Check sheet for the modelled part. Datum: model origin and axes. Units: mm. A direction names the side the tool comes from. Give positions to 0.01 mm unless a question says otherwise; leave off trailing zeros. Loops run counter-clockwise (first coordinate to the right, second up) from the corner with the lowest first, then second, coordinate; pieces in that order, holes last.
```python
from build123d import *

# Parameters (mm, degrees)
SKETCH1_W           = 104.5
SKETCH1_H           = 125.5
BOSS_EXTRUDE1_DEPTH = 4
FILLET1_R           = 5.25
EXTRUDE_THIN1_START = 11
EXTRUDE_THIN1_DEPTH = 11
CUT_EXTRUDE2_REACH  = 138.387
SKETCH6_R           = 1.5
SKETCH8_W           = 10
SKETCH8_H           = 11
BOSS_EXTRUDE2_DEPTH = 4.5
CHAMFER2_SIZE       = 4.5
SKETCH5_R           = 1.9
CUT_EXTRUDE3_DEPTH  = 164.998475603
SKETCH10_R          = 2.45
CUT_EXTRUDE4_DEPTH  = 5
SKETCH2_R           = 5.5
BOSS_EXTRUDE3_DEPTH = 8
CUT_EXTRUDE5_DEPTH  = 137.386628743
SKETCH13_R          = 1.75
CUT_EXTRUDE6_DEPTH  = 137.386628743
CHAMFER3_SIZE       = 4
SKETCH14_R          = 1.75
CUT_EXTRUDE7_DEPTH  = 137.386628743


with BuildPart() as part:
    # Sketch1 → Boss-Extrude1 (new body)
    with BuildSketch(Plane(origin=(0, 0, 0), x_dir=(1, 0, 0), z_dir=(0, 1, 0))):
        with Locations((0, 62.75)):
            Rectangle(SKETCH1_W, SKETCH1_H)
    extrude(amount=BOSS_EXTRUDE1_DEPTH)

    # Fillet1
    fillet1_edges = [part.edges().sort_by_distance(p)[0] for p in [
        (-52.25, 2, -125.5),
        (52.25, 2, -125.5),
        (52.25, 2, 0),
        (-52.25, 2, 0),
    ]]
    fillet(fillet1_edges, radius=FILLET1_R)

    # Sketch3 → Extrude-Thin1 (add)
    with BuildSketch(Plane(origin=(0, 4, 0), x_dir=(1, 0, 0), z_dir=(0, 1, 0)).offset(EXTRUDE_THIN1_START)):
        with BuildLine():
            Line((47, 125.5), (-47, 125.5))
            ThreePointArc((-47, 125.5), (-50.712310601, 123.962310601), (-52.25, 120.25))
            Line((-52.25, 120.25), (-52.25, 5.25))
            ThreePointArc((-52.25, 5.25), (-50.712310601, 1.537689399), (-47, 0))
            Line((-47, 0), (47, 0))
            ThreePointArc((47, 0), (50.712310601, 1.537689399), (52.25, 5.25))
            Line((52.25, 5.25), (52.25, 120.25))
            ThreePointArc((52.25, 120.25), (50.712310601, 123.962310601), (47, 125.5))
        make_face()
        with BuildLine():
            Line((47, 122.5), (-47, 122.5))
            ThreePointArc((-47, 122.5), (-48.590990258, 121.840990258), (-49.25, 120.25))
            Line((-49.25, 120.25), (-49.25, 5.25))
            ThreePointArc((-49.25, 5.25), (-48.590990258, 3.659009742), (-47, 3))
            Line((-47, 3), (47, 3))
            ThreePointArc((47, 3), (48.590990258, 3.659009742), (49.25, 5.25))
            Line((49.25, 5.25), (49.25, 120.25))
            ThreePointArc((49.25, 120.25), (48.590990258, 121.840990258), (47, 122.5))
        make_face(mode=Mode.SUBTRACT)
    extrude(amount=-EXTRUDE_THIN1_DEPTH)

    # Sketch6 → Cut-Extrude2 (cut, up to next)
    with BuildSketch(Plane(origin=(0, 4, 0), x_dir=(1, 0, 0), z_dir=(0, 1, 0)), mode=Mode.PRIVATE) as cut_extrude2_sk1:
        with Locations(Location((-37.5, 110.75, 0), (0, 0, 270))):
            Circle(SKETCH6_R)
    cut_extrude2_tool1 = extrude(cut_extrude2_sk1.sketch, amount=-CUT_EXTRUDE2_REACH, mode=Mode.PRIVATE) & part.part
    # Sketch6 → Cut-Extrude2 (cut, up to next)
    with BuildSketch(Plane(origin=(0, 4, 0), x_dir=(1, 0, 0), z_dir=(0, 1, 0)), mode=Mode.PRIVATE) as cut_extrude2_sk2:
        with Locations(Location((37.5, 110.75, 0), (0, 0, 270))):
            Circle(SKETCH6_R)
    cut_extrude2_tool2 = extrude(cut_extrude2_sk2.sketch, amount=-CUT_EXTRUDE2_REACH, mode=Mode.PRIVATE) & part.part
    # Sketch6 → Cut-Extrude2 (cut, up to next)
    with BuildSketch(Plane(origin=(0, 4, 0), x_dir=(1, 0, 0), z_dir=(0, 1, 0)), mode=Mode.PRIVATE) as cut_extrude2_sk3:
        with Locations(Location((37.5, 35.75, 0), (0, 0, 270))):
            Circle(SKETCH6_R)
    cut_extrude2_tool3 = extrude(cut_extrude2_sk3.sketch, amount=-CUT_EXTRUDE2_REACH, mode=Mode.PRIVATE) & part.part
    # Sketch6 → Cut-Extrude2 (cut, up to next)
    with BuildSketch(Plane(origin=(0, 4, 0), x_dir=(1, 0, 0), z_dir=(0, 1, 0)), mode=Mode.PRIVATE) as cut_extrude2_sk4:
        with Locations(Location((-37.5, 35.75, 0), (0, 0, 270))):
            Circle(SKETCH6_R)
    cut_extrude2_tool4 = extrude(cut_extrude2_sk4.sketch, amount=-CUT_EXTRUDE2_REACH, mode=Mode.PRIVATE) & part.part
    add(cut_extrude2_tool1.solids().sort_by_distance((-37.5, 4, -110.75))[0], mode=Mode.SUBTRACT)
    add(cut_extrude2_tool2.solids().sort_by_distance((37.5, 4, -110.75))[0], mode=Mode.SUBTRACT)
    add(cut_extrude2_tool3.solids().sort_by_distance((37.5, 4, -35.75))[0], mode=Mode.SUBTRACT)
    add(cut_extrude2_tool4.solids().sort_by_distance((-37.5, 4, -35.75))[0], mode=Mode.SUBTRACT)

    # Sketch8 → Boss-Extrude2 (add)
    with BuildSketch(Plane(origin=(-49.25, 0, 0), x_dir=(0, 0, -1), z_dir=(1, 0, 0))):
        with Locations((28.55, 9.5)):
            Rectangle(SKETCH8_W, SKETCH8_H)
        with Locations((108.55, 9.5)):
            Rectangle(SKETCH8_W, SKETCH8_H)
    boss_extrude2 = extrude(amount=BOSS_EXTRUDE2_DEPTH)

    # Mirror4: Boss-Extrude2 across plane
    add(boss_extrude2.mirror(Plane(origin=(0, 0, 0), x_dir=(0, 0, 1), z_dir=(1, 0, 0))))

    # Chamfer2
    chamfer2_edges = [part.edges().sort_by_distance(p)[0] for p in [
        (-49.25, 9.5, -113.55),
        (-49.25, 9.5, -103.55),
        (-49.25, 9.5, -33.55),
        (-49.25, 9.5, -23.55),
        (49.25, 9.5, -113.55),
        (49.25, 9.5, -103.55),
        (49.25, 9.5, -23.55),
        (49.25, 9.5, -33.55),
    ]]
    chamfer(chamfer2_edges, length=CHAMFER2_SIZE - 0.0001)  # a hair under: the kernel refuses the full size

    # Sketch5 → Cut-Extrude3 (cut, through all)
    with BuildSketch(Plane.ZY.offset(52.25)):
        with Locations((-108.55, 10)):
            Circle(SKETCH5_R)
        with Locations((-28.55, 10)):
            Circle(SKETCH5_R)
    extrude(amount=-CUT_EXTRUDE3_DEPTH, mode=Mode.SUBTRACT)

    # Sketch10 → Cut-Extrude4 (cut)
    with BuildSketch(Plane(origin=(-44.75, 0, 0), x_dir=(0, 0, -1), z_dir=(1, 0, 0))):
        with Locations((28.55, 10)):
            Circle(SKETCH10_R)
        with Locations((108.55, 10)):
            Circle(SKETCH10_R)
    cut_extrude4 = extrude(amount=-CUT_EXTRUDE4_DEPTH, mode=Mode.SUBTRACT)

    # Sketch2 → Boss-Extrude3 (add)
    with BuildSketch(Plane.XZ):
        with Locations(Location((-37.5, -14.75, 0), (0, 0, 90))):
            Circle(SKETCH2_R)
        with Locations(Location((37.5, -14.75, 0), (0, 0, 90))):
            Circle(SKETCH2_R)
        with Locations(Location((-22.5, -110.5, 0), (0, 0, 90))):
            Circle(SKETCH2_R)
        with Locations(Location((22.5, -110.5, 0), (0, 0, 90))):
            Circle(SKETCH2_R)
    extrude(amount=-BOSS_EXTRUDE3_DEPTH)

    # Sketch12 → Cut-Extrude5 (cut, through all)
    with BuildSketch(Plane(origin=(0, 4, 0), x_dir=(1, 0, 0), z_dir=(0, 1, 0))):
        Polygon((-34.324573519, 14.75), (-35.91228676, 17.5), (-39.08771324, 17.5), (-40.675426481, 14.75), (-39.08771324, 12), (-35.91228676, 12), align=None)
        Polygon((35.91228676, 12), (34.324573519, 14.75), (35.91228676, 17.5), (39.08771324, 17.5), (40.675426481, 14.75), (39.08771324, 12), align=None)
        Polygon((25.675426481, 110.5), (24.08771324, 107.75), (20.91228676, 107.75), (19.324573519, 110.5), (20.91228676, 113.25), (24.08771324, 113.25), align=None)
        Polygon((-19.324573519, 110.5), (-20.91228676, 113.25), (-24.08771324, 113.25), (-25.675426481, 110.5), (-24.08771324, 107.75), (-20.91228676, 107.75), align=None)
    extrude(amount=CUT_EXTRUDE5_DEPTH, mode=Mode.SUBTRACT)

    # Sketch13 → Cut-Extrude6 (cut, through all)
    with BuildSketch(Plane(origin=(0, 4, 0), x_dir=(1, 0, 0), z_dir=(0, 1, 0))):
        with Locations(Location((37.5, 14.75, 0), (0, 0, 270))):
            Circle(SKETCH13_R)
        with Locations(Location((-37.5, 14.75, 0), (0, 0, 270))):
            Circle(SKETCH13_R)
        with Locations(Location((-22.5, 110.5, 0), (0, 0, 270))):
            Circle(SKETCH13_R)
        with Locations(Location((22.5, 110.5, 0), (0, 0, 270))):
            Circle(SKETCH13_R)
    extrude(amount=-CUT_EXTRUDE6_DEPTH, mode=Mode.SUBTRACT)

    # Chamfer3
    chamfer3_edges = [part.edges().sort_by_distance(p)[0] for p in [
        (-37.5, 4, -20.25),
        (37.5, 4, -20.25),
    ]]
    chamfer(chamfer3_edges, length=CHAMFER3_SIZE - 0.0001)  # a hair under: the kernel refuses the full size

    # Sketch14 → Cut-Extrude7 (cut, through all)
    with BuildSketch(Plane(origin=(0, 4, 0), x_dir=(1, 0, 0), z_dir=(0, 1, 0))):
        with Locations(Location((-42.25, 96.25, 0), (0, 0, 270))):
            Circle(SKETCH14_R)
        with Locations(Location((19.75, 96.25, 0), (0, 0, 270))):
            Circle(SKETCH14_R)
        with Locations(Location((19.75, 44.25, 0), (0, 0, 270))):
            Circle(SKETCH14_R)
        with Locations(Location((-42.25, 44.25, 0), (0, 0, 270))):
            Circle(SKETCH14_R)
    extrude(amount=-CUT_EXTRUDE7_DEPTH, mode=Mode.SUBTRACT)

    # Mirror5: Cut-Extrude4 across plane
    add(cut_extrude4.mirror(Plane(origin=(0, 0, 0), x_dir=(0, 0, 1), z_dir=(1, 0, 0))), mode=Mode.SUBTRACT)


solid = part.part
```
(1) Access from +Z, -Z, +X, -X, +Y, -Y to the whole of each face (thin tool, end or side, straight path). Record for faces 4 (the face through (-1, 0, -64)), 5 (the face through (44.75, 7, -28)).
(2) Section check A-A on x = 37.5. Give the number of separate pieces and of enclosed holes in the cut face, plus the area to 3 significant figures.
(3) Section check C-C on x = -22.5. Record the boundary of the cut face in (y, z), plus the area to 3 significant figures.
(4) Section check B-B on z = -28.55. Record the boundary of the cut face in (x, y).
(5) Section check D-D on x = -10.5. Record the boundary of the cut face in (y, z), plus the area to 3 significant figures.
(6) Material ranges on line 1 (Z direction, x = 22.5, y = 6.25); line 2 (X direction, y = 1.85, z = -44.25); line 3 (X direction, y = 0.9, z = -110.5), recorded low to high.
(7) Release check for a two-part mould opening along Y. For faces 1 (the face through (51, 8.3, -27.7)), 2 (the face through (-49.25, 10, -69)), 3 (the face through (-36, 4, -16)) record: pulls with the +Y half, pulls with the -Y half, needs draft (parallel to the pull), parting line crosses it, or undercut.
(8) Gauge pin test, flat ends, axial feed: pin 1 Ø1 at (x, z) = (-40.5, -46.5) entering from -Y; pin 2 Ø3 at (x, z) = (17, -45) entering from +Y. Record the tip position at first contact, or that the pin passes through.
Computed values:
1. face 4: +Z, -Z, +X, -X, -Y
1. face 5: +Y
2. separate pieces: 4
2. enclosed holes: 0
2. area: 568 mm2
3. outline: (0, -125.5) - (15, -125.5) - (15, -122.5) - (4, -122.5) - (4, -116) - (8, -116) - (8, -113.25) - (4, -113.25) - (4, -112.25) - (0, -112.25) - close; (0, -108.75) - (4, -108.75) - (4, -107.75) - (8, -107.75) - (8, -105) - (4, -105) - (4, -3) - (15, -3) - (15, 0) - (0, 0) - close
3. area: 576 mm2
4. outline: (-52.25, 0) - (52.25, 0) - (52.25, 8.1) - (49.75, 8.1) - (49.75, 7.55) - (44.75, 7.55) - (44.75, 4) - (-44.75, 4) - (-44.75, 7.55) - (-49.75, 7.55) - (-49.75, 8.1) - (-52.25, 8.1) - close; (-52.25, 11.9) - (-49.75, 11.9) - (-49.75, 12.45) - (-44.75, 12.45) - (-44.75, 15) - (-52.25, 15) - close; (44.75, 12.45) - (49.75, 12.45) - (49.75, 11.9) - (52.25, 11.9) - (52.25, 15) - (44.75, 15) - close
5. outline: (0, -125.5) - (15, -125.5) - (15, -122.5) - (4, -122.5) - (4, -3) - (15, -3) - (15, 0) - (0, 0) - close
5. area: 568 mm2
6. line 1: z = -125.5 to -122.5, -116 to -113.25, -107.75 to -105, -3 to 0
6. line 2: x = -52.25 to -44, -40.5 to 18, 21.5 to 52.25
6. line 3: x = -52.25 to -38.98, -36.02 to -24.25, -20.75 to 20.75, 24.25 to 36.02, 38.98 to 52.25
7. face 1: undercut
7. face 2: needs draft
7. face 3: pulls with the +Y half
8. pin 1: stops at y = 0
8. pin 2: stops at y = 4
